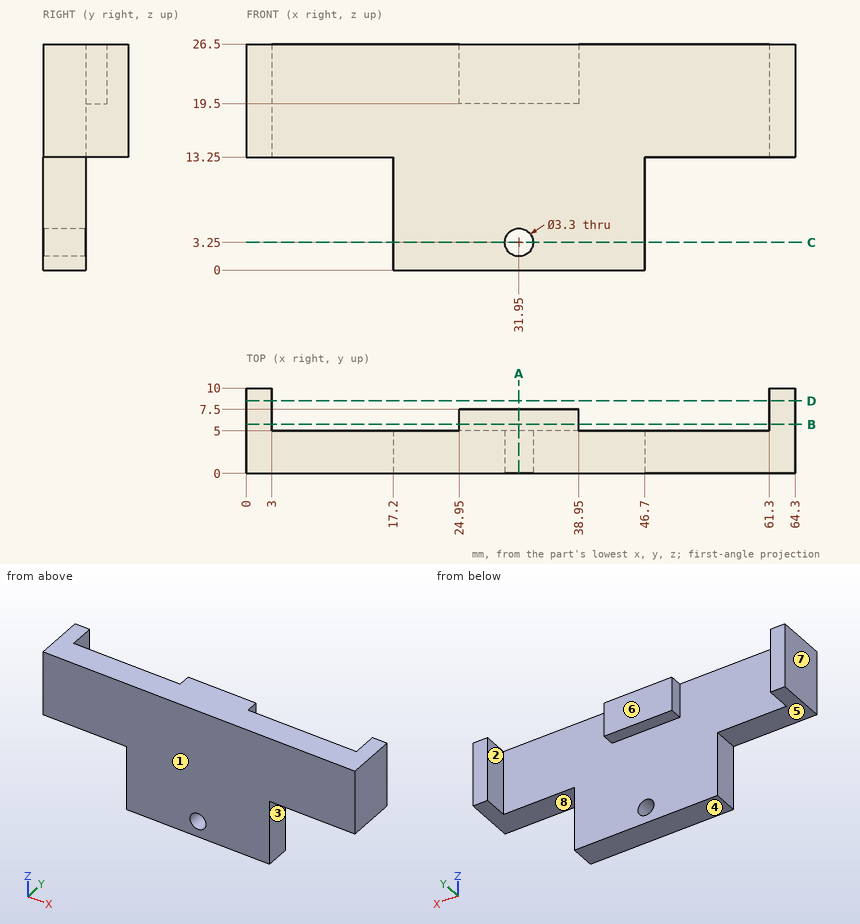
Can you work these out from the drawing? Everything is in mm from the part's minimum corner. A direction names the side the tool comes from. Round coordinates to 2 decimals unless told otherwise and drop trailing zeros. Write each loop counter-clockwise with the first axis right and the second up, starting at its lowest first coordinate (ties: lowest second). Pieces come first, ordered by that corner, then holes. Notation, with made-up numbers: (42, 34) - (100, 34) arc R12 cw to (100, 57) - close; hole circle Ø8 at (20.25, 65.25). An arc over 180 degrees is marked (long way). Use a Markdown table: item, result.
Q1. Please list where these lines run through material, in increasing order: L1, parallel to X at y = 6, z = 21; L2, parallel to X at y = 1.65, z = 3.25; L3, parallel to X at y = 6.25, z = 16.5.
Output values:
| item | result |
|---|---|
| L1 | 0 to 3, 24.95 to 38.95, 61.3 to 64.3 |
| L2 | 17.2 to 30.3, 33.6 to 46.7 |
| L3 | 0 to 3, 61.3 to 64.3 |
Q2. I want a section at A-A (x = 31.95). List the corners of the cut face in (y, z) for me, plus the area to 4 significant figures.
Output values:
| item | result |
|---|---|
| outline | (0, 0) - (5, 0) - (5, 1.6) - (0, 1.6) - close; (0, 4.9) - (5, 4.9) - (5, 19.5) - (7.5, 19.5) - (7.5, 26.5) - (0, 26.5) - close |
| area | 133.5 mm2 |
Q3. I want a section at C-C (z = 3.25). List the corners of the cut face in (x, y) for me, plus the area to 3 significant figures.
Output values:
| item | result |
|---|---|
| outline | (17.2, 0) - (30.3, 0) - (30.3, 5) - (17.2, 5) - close; (33.6, 0) - (46.7, 0) - (46.7, 5) - (33.6, 5) - close |
| area | 131 mm2 |
Q4. I want a section at B-B (y = 5.75). List the corners of the cut face in (x, z) for me, plus the area to 4 significant figures.
Output values:
| item | result |
|---|---|
| outline | (0, 13.25) - (3, 13.25) - (3, 26.5) - (0, 26.5) - close; (24.95, 19.5) - (38.95, 19.5) - (38.95, 26.5) - (24.95, 26.5) - close; (61.3, 13.25) - (64.3, 13.25) - (64.3, 26.5) - (61.3, 26.5) - close |
| area | 177.5 mm2 |
Q5. Thinking about a two-plate mould opening in X: for the marked faces 6, 7 and 8, which applies, released by +X, released by -X, zero draft, split by the parting line, or undercut?
Output values:
| item | result |
|---|---|
| face 6 | undercut |
| face 7 | released by -X |
| face 8 | zero draft |
Q6. For pin 1 (2 mm diameter, centred on x = 31.95, z = 3.25, fed in from -Y); pin 2 (4 mm diameter, centred on y = 3, z = 7, fed in from +X); pin 3 (5.5 mm diameter, centred on y = 3.5, z = 6.5, fed in from -X); pin 4 (5.5 mm diameter, centred on x = 34.5, z = 21.5, fed in from +Y), each with a flat end and sliding along its axis, tell me the tip position at first contact or that it passes through.
Output values:
| item | result |
|---|---|
| pin 1 | through |
| pin 2 | x = 46.7 |
| pin 3 | x = 17.2 |
| pin 4 | y = 7.5 |
Q7. For the marked faces 1, 2, 3, 4 and 5, which set-ups out of +Z, -Z, +X, -X, +Y, -Y let a thin tool reach every point of the face, with its end or its side?
Output values:
| item | result |
|---|---|
| face 1 | +Z, -Z, +X, -X, -Y |
| face 2 | +Z, -Z, +Y |
| face 3 | -Z, +X, +Y, -Y |
| face 4 | -Z, +X, -X, +Y, -Y |
| face 5 | -Z, -X, +Y, -Y |
Q8. I want a section at D-D (y = 8.5). List the corners of the cut face in (x, z) for me.
Output values:
| item | result |
|---|---|
| outline | (0, 13.25) - (3, 13.25) - (3, 26.5) - (0, 26.5) - close; (61.3, 13.25) - (64.3, 13.25) - (64.3, 26.5) - (61.3, 26.5) - close |
